Verification items for this drawing (mm, ordinates from the low corner). A direction names the side the tool comes from. Round coordinates to 2 decimals unless told otherwise and drop trailing zeros. Write each loop counter-clockwise with the first axis right and the second up, starting at its lowest first coordinate (ties: lowest second). Pieces come first, ordered by that corner, then holes. Notation, with made-up numbers: (52, -6.5) -> (56, -6.5) arc R19 cw to (56, 6.5) -> close; hole circle Ø7 at (48.25, 34). An arc over 180 degrees is marked (long way). Put each result on its own line as item: value. Start each with the question number.
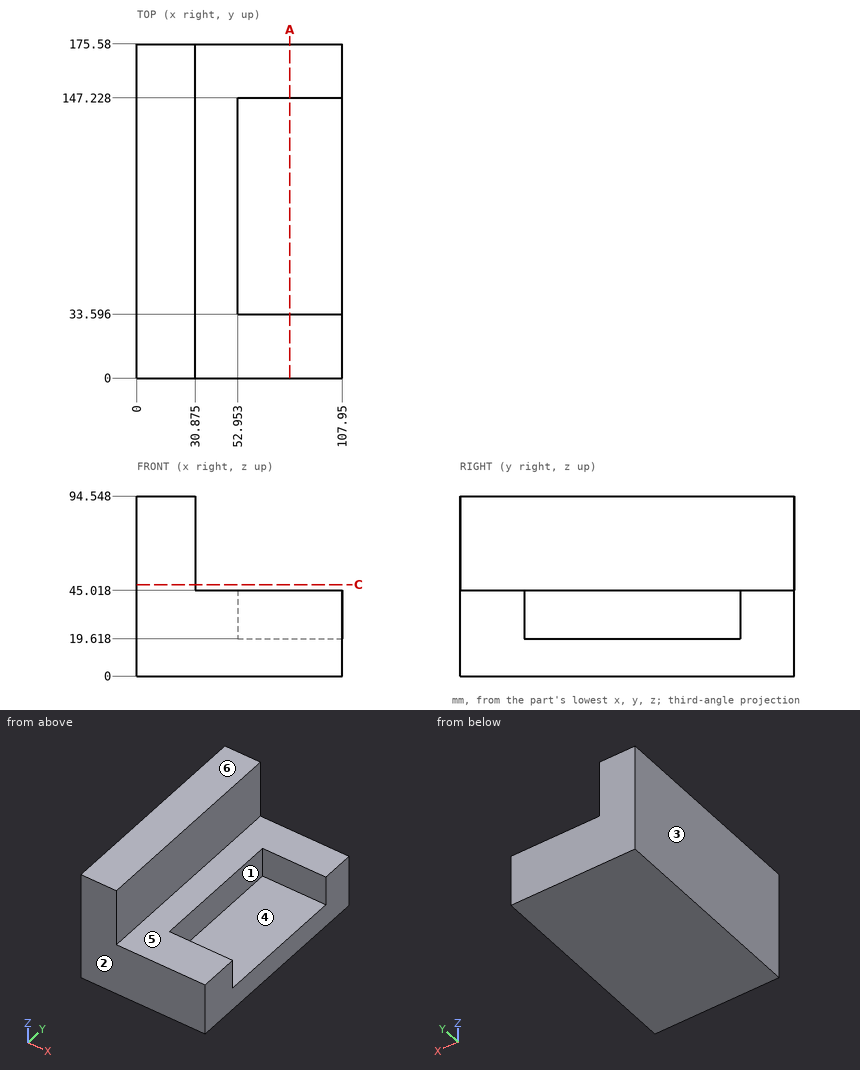
(1) Go/stop test with flat-tipped pins: pin 1 Ø20.5 at (y, z) = (93.5, 32.5) entering from +X; pin 2 Ø10 at (y, z) = (136.5, 72) entering from -X; pin 3 Ø3 at (x, y) = (60, 41) entering from +Z. Record where each tip stops, or that it passes through.
(2) Sectioned sample at A-A (x = 80.5). Record the cut outline in (y, z), and give its area (3 significant figures).
(3) Mould release check, pull along Y, two halves, no side actions. Record for the marked faces 1, 2 and 3: +Y half, -Y half, draft (parallel to the pull), parting line (faces both ways), or undercut.
(4) Material ranges on L1, parallel to Y at x = 78, z = 23; L2, parallel to X at y = 166.5, z = 84 (1 decimal); L3, parallel to X at y = 128, z = 37, recorded low to high. Write a range as from..to.
(5) Sectioned sample at C-C (z = 48). Record the cut outline in (x, y) (1 decimal), and give its area (3 significant figures).
(6) Set-up check for the marked faces 4, 5 and 6: record each of +Z, -Z, +X, -X, +Y, -Y from which the full face is reachable in a straight line by a thin tool's end or side.
Found:
1. pin 1: x = 52.95
1. pin 2: x = 0
1. pin 3: z = 19.62
2. outline: (0, 0) -> (175.58, 0) -> (175.58, 45.02) -> (147.23, 45.02) -> (147.23, 19.62) -> (33.6, 19.62) -> (33.6, 45.02) -> (0, 45.02) -> close
2. area: 5,020 mm2
3. face 1: undercut
3. face 2: -Y half
3. face 3: draft
4. L1: 0..33.6, 147.23..175.58
4. L2: 0..30.9
4. L3: 0..52.95
5. outline: (0, 0) -> (30.9, 0) -> (30.9, 175.6) -> (0, 175.6) -> close
5. area: 5,420 mm2
6. face 4: +Z, +X
6. face 5: +Z, +X, +Y, -Y
6. face 6: +Z, +X, -X, +Y, -Y
